Source: three-view drawing plus pictorial views. Frame: mm from the lowest corner of the part. A direction names the side the tool comes from. Give positions to 0.01 mm unless a question says otherwise; leave off trailing zeros. Write each loop counter-clockwise with the first axis right and the second up, starting at its lowest first coordinate (ties: lowest second). Pieces come first, ordered by that corner, then holes.
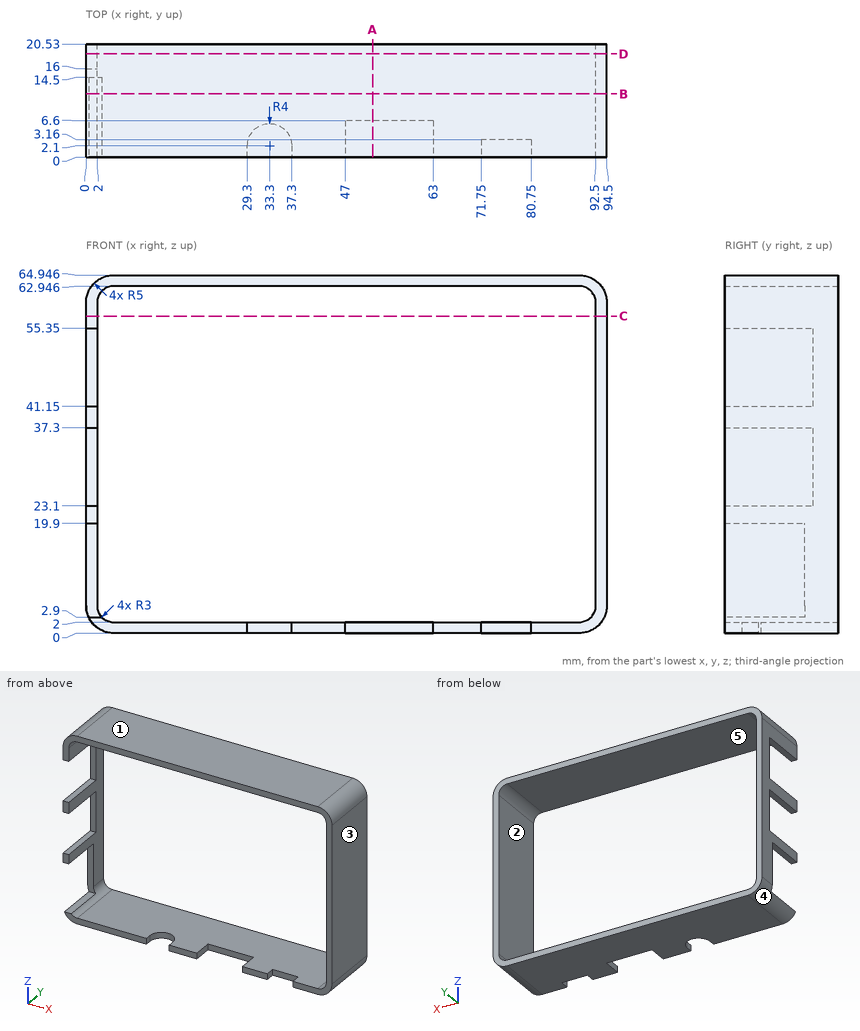
Q1. Section C-C on z = 57.5. Output: boundary loops of the cut face in (x, y).
Filled sheet:
outline: (0, 0) - (2, 0) - (2, 20.53) - (0, 20.53) - close; (92.5, 0) - (94.5, 0) - (94.5, 20.53) - (92.5, 20.53) - close
Q2. Pin query (flat end, axial travel): P1, Ø2.5, axis at x = 1.5, y = 4, coming from the +Z side; P2, Ø2, axis at x = 76.5, z = 0.5, coming from the -Y side; P3, Ø0.6, axis at y = 3, z = 0.5, coming from the -X side. Return the tip coordinate at first contact, or that it passes through.
Filled sheet:
P1: stops at z = 64.41
P2: stops at y = 3.16
P3: stops at x = 2.29
Q3. Access query for the marked faces 4 and 5. Directions: +Z, -Z, +X, -X, +Y, -Y. A direction counts if a zero-diameter tool reaches every point of the face in a straight line with its end or side. Return the directions, or none.
Filled sheet:
face 4: -Z, -X, +Y, -Y
face 5: +Y, -Y
Q4. Section D-D on y = 18.75. Output: boundary loops of the cut face in (x, z), plus the area to 3 significant figures.
Filled sheet:
outline: (0, 5) arc R5 ccw to (5, 0) - (89.5, 0) arc R5 ccw to (94.5, 5) - (94.5, 59.95) arc R5 ccw to (89.5, 64.95) - (5, 64.95) arc R5 ccw to (0, 59.95) - close; hole (2, 5) arc R3 ccw to (5, 2) - (89.5, 2) arc R3 ccw to (92.5, 5) - (92.5, 59.95) arc R3 ccw to (89.5, 62.95) - (5, 62.95) arc R3 ccw to (2, 59.95) - close
area: 608 mm2
Q5. Section A-A on x = 52. Output: boundary loops of the cut face in (y, z).
Filled sheet:
outline: (0, 62.95) - (20.53, 62.95) - (20.53, 64.95) - (0, 64.95) - close; (6.6, 0) - (20.53, 0) - (20.53, 2) - (6.6, 2) - close
Q6. Pull-direction query (X, two-part tool) for the marked faces 1, 2 and 3; classes: released by +X, released by -X, zero draft, split by the parting line, or undercut.
Filled sheet:
face 1: zero draft
face 2: undercut
face 3: released by +X
Q7. Section B-B on y = 11.5. Output: boundary loops of the cut face in (x, z), plus the area to 3 significant figures.
Filled sheet:
outline: (0, 19.9) - (2, 19.9) - (2, 23.1) - (0, 23.1) - close; (0, 37.3) - (2, 37.3) - (2, 41.15) - (0, 41.15) - close; (0, 55.35) - (2, 55.35) - (2, 59.95) arc R3 cw to (5, 62.95) - (89.5, 62.95) arc R3 cw to (92.5, 59.95) - (92.5, 5) arc R3 cw to (89.5, 2) - (5, 2) arc R3 cw to (2.86, 2.9) - (0.46, 2.9) arc R5 ccw to (5, 0) - (89.5, 0) arc R5 ccw to (94.5, 5) - (94.5, 59.95) arc R5 ccw to (89.5, 64.95) - (5, 64.95) arc R5 ccw to (0, 59.95) - close
area: 517 mm2
Q8. Ray query, line 1 along X through (y, z) = (19.5, 12); line 2 along Z through (x, y) = (66, 5.25); line 3 along X through (y, z) = (7.5, 12). Return the intervals inside material, ascending.
Filled sheet:
line 1: x = 0 to 2, 92.5 to 94.5
line 2: z = 0 to 2, 62.95 to 64.95
line 3: x = 92.5 to 94.5
